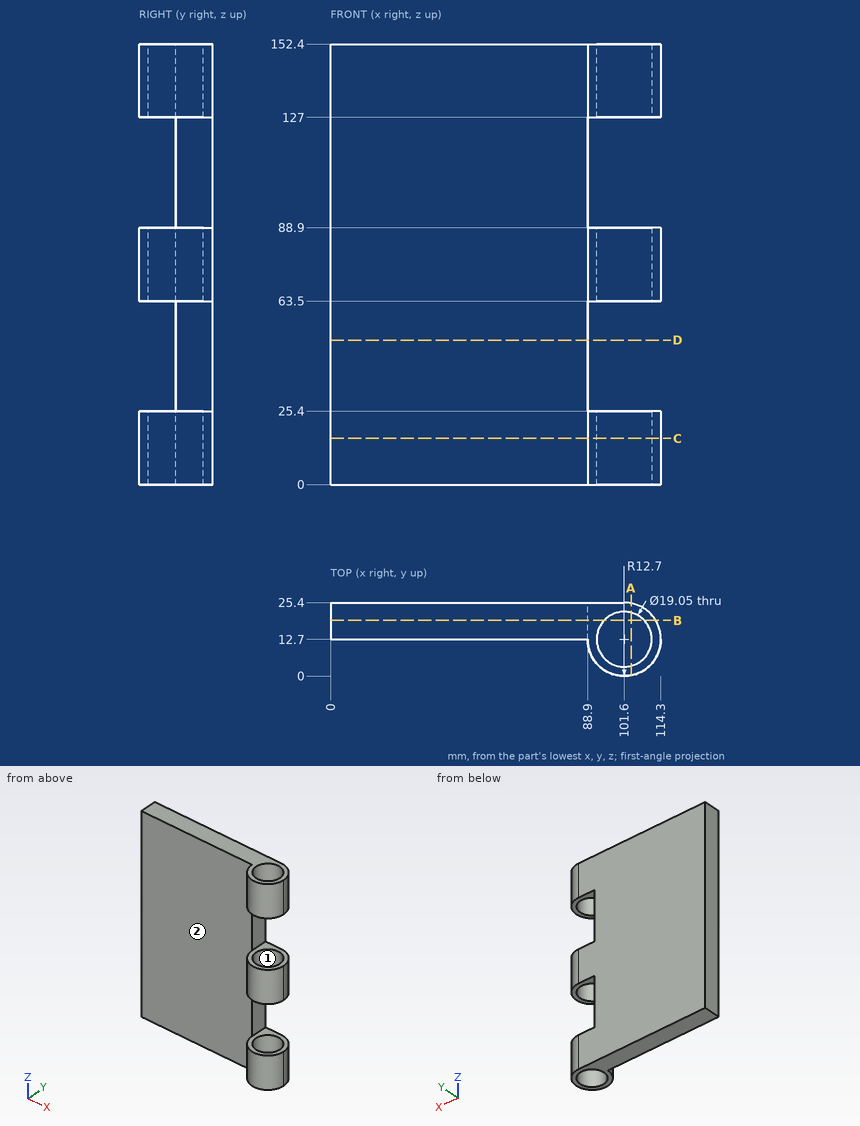
Input: dimensioned drawing with shaded views. Units: mm. Origin: part minimum x, y, z. A direction names the side the tool comes from. Give positions to 0.01 mm unless a question says otherwise; leave off trailing zeros. Order: outer loops, then holes, each group sorted by start corner. A loop starts at its lowest first (then second) coordinate and runs counter-clockwise, first axis right, second up.
(1) Section query C-C (z = 16). Return the cut outline in (x, y) (3 decimals).
(2) Section query A-A (x = 104). Return the cut outline in (y, z).
(3) Section query B-B (y = 19.25). Return the cut outline in (x, z), plus the area to 3 significant figures.
(4) Material intervals for line 1 along Y through (x, z) = (101.6, 15.25) (3 decimals); line 2 along Y through (x, z) = (44.5, 56); line 3 along Y through (x, z) = (100, 88), sorted ascending.
(5) Contact query for flat-ended pins moving along their axis: P1, Ø5, axis at y = 10.5, z = 69.5, coming from the +X side; P2, Ø5, axis at x = 53, z = 40.5, coming from the -Y side; P3, Ø3, axis at y = 10.5, z = 78, coming from the -X side; P4, Ø4, axis at y = 21.5, z = 49.5, coming from the +X side. Output: stop coordinate, or through.
(6) Section query D-D (z = 50). Return the cut outline in (x, y), plus the area to 3 significant figures.
(7) Access query for the marked faces 1 and 2. Directions: +Z, -Z, +X, -X, +Y, -Y. A direction counts if a zero-diameter tool reaches every point of the face in a straight line with its end or side. Return the directions, or none.
Outcome:
1. outline: (0, 12.7) - (88.9, 12.7) arc R12.7 ccw (long way) to (101.6, 25.4) - (0, 25.4) - close; hole circle Ø19.05 at (101.6, 12.7)
2. outline: (0.23, 0) - (3.48, 0) - (3.48, 25.4) - (0.23, 25.4) - close; (0.23, 63.5) - (3.48, 63.5) - (3.48, 88.9) - (0.23, 88.9) - close; (0.23, 127) - (3.48, 127) - (3.48, 152.4) - (0.23, 152.4) - close; (21.92, 0) - (25.17, 0) - (25.17, 25.4) - (21.92, 25.4) - close; (21.92, 63.5) - (25.17, 63.5) - (25.17, 88.9) - (21.92, 88.9) - close; (21.92, 127) - (25.17, 127) - (25.17, 152.4) - (21.92, 152.4) - close
3. outline: (0, 0) - (94.68, 0) - (94.68, 25.4) - (88.9, 25.4) - (88.9, 63.5) - (94.68, 63.5) - (94.68, 88.9) - (88.9, 88.9) - (88.9, 127) - (94.68, 127) - (94.68, 152.4) - (0, 152.4) - close; (108.52, 0) - (112.48, 0) - (112.48, 25.4) - (108.52, 25.4) - close; (108.52, 63.5) - (112.48, 63.5) - (112.48, 88.9) - (108.52, 88.9) - close; (108.52, 127) - (112.48, 127) - (112.48, 152.4) - (108.52, 152.4) - close
3. area: 14,300 mm2
4. line 1: y = 0 to 3.175, 22.225 to 25.4
4. line 2: y = 12.7 to 25.4
4. line 3: y = 0.1 to 3.31, 22.09 to 25.4
5. P1: stops at x = 114.3
5. P2: stops at y = 12.7
5. P3: stops at x = 88.92
5. P4: stops at x = 88.9
6. outline: (0, 12.7) - (88.9, 12.7) - (88.9, 25.4) - (0, 25.4) - close
6. area: 1,130 mm2
7. face 1: +Z, -Z
7. face 2: +Z, -Z, -X, -Y
